Autodesk Inventor part; units mm, degrees
ref_plane "YZ Plane" through (0, 0, 0) normal (1, 0, 0) x (0, 1, 0)
ref_plane "XZ Plane" through (0, 0, 0) normal (0, 1, 0) x (-1, 0, 0)
ref_plane "XY Plane" through (0, 0, 0) normal (0, 0, 1) x (1, 0, 0)
sketch "Sketch1" plane through (0, 0, 0) normal (0, 1, 0) x (-1, 0, 0)
  line L0 (-55, 100) -> (55, 100)
  line L1 (55, 100) -> (55, -100)
  line L2 (55, -100) -> (-55, -100)
  line L3 (-55, -100) -> (-55, 100)
  line L4 (-55, 100) -> (55, -100) construction
  line L5 (55, 100) -> (-55, -100) construction
  point P0 (0, 0)
  dimension "d0" = 110
  dimension "d1" = 200
extrude "Extrusion1" add sketch "Sketch1" along normal blind 22
sketch "Sketch2" plane through (0, 22, 0) normal (0, 1, 0) x (1, 0, 0)
  line L0 (55, -100) -> (55, 100) construction
  line L1 (55, 100) -> (40, 100) construction
  line L2 (55, 100) -> (-55, 100) construction
  line L3 (55, 100) -> (70, 100) construction
  line L4 (40, 100) -> (-10, 100)
  line L5 (-10, 100) -> (-10, -20)
  line L6 (-10, -20) -> (40, -20)
  line L7 (40, -20) -> (40, 100)
  point P0 (0, 0)
  dimension "d4" = 15
  dimension "d5" = 180
  dimension "d6" = 50
  dimension "d7" = 120
sketch "Sketch3" plane through (0, 0, 0) normal (0, -1, 0) x (1, 0, 0)
  line L0 (-51, 96) -> (51, 96)
  line L1 (51, 96) -> (51, -96)
  line L2 (51, -96) -> (-51, -96)
  line L3 (-51, -96) -> (-51, 96)
  line L4 (-51, 96) -> (51, -96) construction
  line L5 (51, 96) -> (-51, -96) construction
  point P0 (0, 0)
  dimension "d8" = 102
  dimension "d9" = 192
extrude "Extrusion2" cut sketch "Sketch3" against normal blind 18
extrude "Extrusion3" cut sketch "Sketch2" against normal up to surface (22 mm away)
sketch "Sketch4" plane through (0, 22, 0) normal (0, 1, 0) x (1, 0, 0)
  line L0 (40, -20) -> (-10, -20)
  line L1 (40, -20) -> (-40, -20)
  line L2 (-40, -20) -> (-40, -85)
  line L3 (-40, -85) -> (40, -85)
  line L4 (40, -85) -> (40, -20)
  point P0 (0, 0)
  dimension "d14" = 80
  dimension "d15" = 65
extrude "Extrusion4" cut sketch "Sketch4" against normal blind 13
sketch "Sketch6" plane through (0, 22, 0) normal (0, 1, 0) x (1, 0, 0)
  line L0 (40, 100) -> (40, -85)
  line L1 (40, -85) -> (-40, -85)
  line L2 (-40, -85) -> (-40, -20)
  line L3 (-40, -20) -> (-10, -20)
  line L4 (-10, -20) -> (-10, 100)
  line L5 (-10, 100) -> (-55, 100)
  line L6 (-55, 100) -> (-55, -100)
  line L7 (-55, -100) -> (55, -100)
  line L8 (55, -100) -> (55, 100)
  line L9 (55, 100) -> (40, 100)
  line L10 (-55, 100) -> (-55, 63) construction
  line L11 (-55, 100) -> (-18, 100) construction
  line L12 (-55, 63) -> (-45, 63) construction
  circle A0 centre (-45, 63) radius 2.5
  line L13 (55, 100) -> (55, -100) construction
  line L14 (55, 100) -> (55, 63) construction
  line L15 (55, 100) -> (92, 100) construction
  line L16 (55, 63) -> (45, 63) construction
  circle A1 centre (45, 63) radius 2.5
  point P0 (0, 0)
  dimension "d24" = 37
  dimension "d25" = 90
  dimension "d26" = 10
  dimension "d27" = 90
  dimension "d28" = 5
  dimension "d29" = 37
  dimension "d30" = 90
  dimension "d31" = 10
  dimension "d32" = 90
  dimension "d33" = 5
extrude "Extrusion6" cut sketch "Sketch6" against normal blind 10 contours A0 | A1
sketch "Sketch8" plane through (0, 18, 0) normal (0, -1, 0) x (1, 0, 0)
  line L0 (51, 96) -> (51, -96) construction
  line L1 (51, 96) -> (35, 96) construction
  line L2 (-51, 96) -> (51, 96) construction
  line L3 (51, 96) -> (67, 96) construction
  line L4 (35, 96) -> (-35, 96)
  line L5 (-35, 96) -> (-35, 85)
  line L6 (-35, 85) -> (35, 85)
  line L7 (35, 85) -> (35, 96)
  point P0 (0, 0)
  dimension "d57" = 16
  dimension "d58" = 180
  dimension "d59" = 70
  dimension "d60" = 11
extrude "Extrusion8" add sketch "Sketch8" along normal blind 13
sketch "Sketch7" plane through (-55, 0, 100) normal (0, 0, 1) x (1, 0, 0)
  line L0 (45, 22) -> (0, 22) construction
  line L1 (0, 22) -> (39.8, 22) construction
  line L2 (39.8, 22) -> (37.3, 17.6699)
  line L3 (39.8, 22) -> (44.8, 22) construction
  line L4 (37.3, 17.6699) -> (47.7, 17.6699)
  line L5 (45, 18) -> (4, 18)
  line L6 (47.7, 17.6699) -> (45.2, 22)
  line L7 (15, 22) -> (45, 22)
  line L8 (45.2, 22) -> (39.8, 22)
  line L9 (0, 22) -> (110, 22)
  line L10 (110, 22) -> (70.2, 22)
  line L11 (110, 22) -> (149.8, 22) construction
  line L12 (70.2, 22) -> (72.7, 17.6699)
  line L13 (72.7, 17.6699) -> (62.3, 17.6699)
  line L14 (15, 18) -> (95, 18)
  line L15 (62.3, 17.6699) -> (64.8, 22)
  line L16 (64.8, 22) -> (70.2, 22)
  point P0 (55, 0)
  dimension "d36" = 39.8
  dimension "d39" = 5
  dimension "d40" = 120
  dimension "d41" = 10.4
  dimension "d42" = 60
  dimension "d43" = 5
  dimension "d44" = 60
  dimension "d45" = 5.4
  dimension "d46" = 120
  dimension "d47" = 39.8
  dimension "d48" = 180
  dimension "d49" = 5
  dimension "d50" = 60
  dimension "d51" = 10.4
  dimension "d52" = 60
  dimension "d53" = 5
  dimension "d54" = 60
extrude "Extrusion7" cut sketch "Sketch7" against normal blind 6 contours L7 L8 L6 L14 L5 L2 | L5 L14 L6 L4 L2 | L9 L12 L14 L15 | L14 L12 L13 L15
sketch "Sketch9" plane through (0, 0, 0) normal (0, -1, 0) x (1, 0, 0)
  line L0 (-10, -100) -> (-10, -96)
  line L1 (-10, -96) -> (-51, -96)
  line L2 (-51, -96) -> (-51, 96)
  line L3 (-51, 96) -> (51, 96)
  line L4 (51, 96) -> (51, -96)
  line L5 (51, -96) -> (40, -96)
  line L6 (40, -96) -> (40, -100)
  line L7 (40, -100) -> (55, -100)
  line L8 (55, -100) -> (55, 100)
  line L9 (55, 100) -> (-55, 100)
  line L10 (-55, 100) -> (-55, -100)
  line L11 (-55, -100) -> (-10, -100)
  line L12 (55, 100) -> (-55, 100)
  line L13 (0, 100) -> (0, 90)
  line L14 (0, 100) -> (10, 100) construction
  line L15 (0, 90) -> (-25, 90)
  line L16 (0, 90) -> (25, 90)
  circle A0 centre (25, 90) radius 1.5
  circle A1 centre (0, 90) radius 1.5
  circle A2 centre (-25, 90) radius 1.5
  point P0 (0, 0)
  dimension "d63" = 10
  dimension "d64" = 90
  dimension "d65" = 25
  dimension "d66" = 180
  dimension "d67" = 3
  dimension "d68" = 3
  dimension "d69" = 3
extrude "Extrusion9" cut sketch "Sketch9" against normal blind 10 contours A0 | A2 | A1 L16 L13 | L13 L15 A1 | L16 A1 L15
sketch "Sketch10" plane through (-55, 0, -100) normal (0, 0, -1) x (-1, 0, 0)
  line L0 (-45, 22) -> (-45, 0)
  line L1 (0, 0) -> (-45, 0)
  line L2 (0, 0) -> (0, 22)
  line L3 (-45, 22) -> (0, 22)
  line L4 (-95, 0) -> (-95, 22)
  line L5 (-110, 22) -> (-95, 22)
  line L6 (-110, 0) -> (-110, 22)
  line L7 (-95, 0) -> (-110, 0)
  line L8 (0, 0) -> (-110, 0)
  line L9 (-110, 0) -> (-110, 22)
  line L10 (-110, 22) -> (0, 22)
  line L11 (0, 22) -> (0, 0)
  point P0 (-55, 0)
extrude "Extrusion11" cut sketch "Sketch10" against normal blind 6 contours L3 L2 L1 L0 | L4 L7 L6 L5
sketch "Sketch11" plane through (0, 22, 0) normal (0, 1, 0) x (1, 0, 0)
  line L0 (-10, -20) -> (-40, -20) construction
  line L1 (-10, -20) -> (-10, -6) construction
  line L2 (-10, 94) -> (-10, -20) construction
  line L3 (-10, -6) -> (-26, -6)
  line L4 (-26, -6) -> (-26, 54)
  line L5 (-26, 54) -> (-10, 54)
  line L6 (-10, 54) -> (-10, -6)
  line L7 (-10, -6) -> (40, -6) construction
  line L8 (40, -85) -> (40, 94) construction
  line L9 (40, -6) -> (50, -6)
  line L10 (50, -6) -> (50, 54)
  line L11 (50, 54) -> (40, 54)
  line L12 (40, 54) -> (40, -6)
  point P0 (0, 0)
  dimension "d77" = 14
  dimension "d78" = 16
  dimension "d79" = 60
  dimension "d80" = 10
  dimension "d81" = 60
extrude "Extrusion12" cut sketch "Sketch11" against normal up to surface (4 mm away)
ref_plane "Work Plane1" through (0, 0, 100) normal (1, 0, 0) x (0, 0, -1)
properties part number "foot_cover_2_bottom"
Here's how the part is built. I have some questions about the finished solid (model axes, mm). A direction names the side the tool comes from. Round coordinates to 2 decimals unless told otherwise and drop trailing zeros. Write each loop counter-clockwise with the first axis right and the second up, starting at its lowest first coordinate (ties: lowest second). Pieces come first, ordered by that corner, then holes. Notation, with made-up numbers: (-18, 69) -> (36, 69) arc R19 ccw to (36, 106) -> close; hole circle Ø10 at (24.5, 80). An arc over 180 degrees is marked (long way). One line per item, written item: value.
1) Suppose I cut it at B-B on x = -29.5. List the corners of the cut face in (y, z) for me, plus the area to 3 significant figures.
Filled sheet:
outline: (0, 96) -> (5, 96) -> (5, 85) -> (22, 85) -> (22, 100) -> (0, 100) -> close; (18, -94) -> (22, -94) -> (22, 20) -> (18, 20) -> close
area: 731 mm2
2) For faces 4 (the face through (-35, 12, 91)), 5 (the face through (-26, 20, -24)), 6 (the face through (-10, 20, -74)), 7 (the face through (-13, 19, 94)), which set-ups out of +Z, -Z, +X, -X, +Y, -Y let a thin tool reach every point of the face, with its end or its side?
Filled sheet:
face 4: -Z, -Y
face 5: +Y, -Y
face 6: -Z, +Y, -Y
face 7: +Z
3) Suppose I cut it at D-D on x = 45. List the corners of the cut face in (y, z) for me.
Filled sheet:
outline: (0, 96) -> (18, 96) -> (18, 6) -> (22, 6) -> (22, 100) -> (0, 100) -> close; (18, -94) -> (22, -94) -> (22, -65.5) -> (18, -65.5) -> close; (18, -60.5) -> (22, -60.5) -> (22, -54) -> (18, -54) -> close
4) I'm going to push flat-ended pins straight in: pin 1 Ø12 at (x, y) = (32, 11) entering from -Z; pin 2 Ø2 at (x, y) = (-11, 20) entering from +Z; pin 3 Ø2.5 at (x, z) = (0, 90) entering from -Y. Where does each tip first touch, or does it pass through?
Filled sheet:
pin 1: stops at z = 85
pin 2: stops at z = 94
pin 3: stops at y = 10
5) We'd pull the mould along Z, two halves only. Please class faces 1 (the face through (53, 16, -94)), 2 (the face through (45, 20, -54)), 3 (the face through (45, 18, 23)): released by +Z, released by -Z, zero draft, split by the parting line, or undercut.
Filled sheet:
face 1: released by -Z
face 2: undercut
face 3: zero draft
6) If I drill on line 1 (Z direction, x = 45, y = 20.3); line 2 (X direction, y = 8.95, z = 90); line 3 (X direction, y = 19.75, z = -63), over which ranges is the centre line in solid material (lowest first)? Write a range as [from, to].
Filled sheet:
line 1: z = [-94, -65.5], [-60.5, -54], [6, 100]
line 2: x = [-55, -51], [-35, -26.5], [-23.5, -1.5], [1.5, 23.5], [26.5, 35], [51, 55]
line 3: x = [-55, -47.5], [-42.5, -10], [40, 42.5], [47.5, 55]
7) Suppose I cut it at C-C on y = 13. List the corners of the cut face in (x, z) for me.
Filled sheet:
outline: (-55, -94) -> (-51, -94) -> (-51, 96) -> (-35, 96) -> (-35, 85) -> (35, 85) -> (35, 96) -> (51, 96) -> (51, -94) -> (55, -94) -> (55, 100) -> (-55, 100) -> close
8) Suppose I cut it at A-A on z = -72.5. List the corners of the cut face in (x, y) for me, plus the area to 3 significant figures.
Filled sheet:
outline: (-55, 0) -> (-51, 0) -> (-51, 18) -> (-10, 18) -> (-10, 22) -> (-55, 22) -> close; (40, 18) -> (51, 18) -> (51, 0) -> (55, 0) -> (55, 22) -> (40, 22) -> close
area: 384 mm2
